Check sheet for the modelled part. Datum: model origin and axes. Units: mm. Coordinates: 2 decimals unless noted, no trailing zeros. Order: outer loops, then holes, each group sorted by start corner. A loop starts at its lowest first (then second) coordinate and runs counter-clockwise, first axis right, second up.
from build123d import *

# Parameters (mm, degrees)
EXTRUDE_1_DEPTH     = 4
SKETCH_3_R          = 2.1
CUT_EXTRUDE_1_DEPTH = 4
SKETCH_4_R          = 10
CUT_EXTRUDE_2_DEPTH = 4
SKETCH_5_W          = 90
SKETCH_5_H          = 5
CUT_EXTRUDE_3_DEPTH = 5
FILLET_1_R          = 5
FILLET_2_R          = 1


with BuildPart() as part:
    # 草图2 → 凸台-拉伸1 (new body)
    with BuildSketch(Plane(origin=(0, 0, 0), x_dir=(1, 0, 0), z_dir=(0, 1, 0))):
        with BuildLine():
            Line((-50, -50), (-50, 50))
            Line((-50, 50), (50, 50))
            Line((50, 50), (50, -50))
            ThreePointArc((50, -50), (0, -100), (-50, -50))
        make_face()
    extrude(amount=EXTRUDE_1_DEPTH)

    # 草图3 → 切除-拉伸1 (cut)
    with BuildSketch(Plane.XZ):
        with Locations(Location((0, 90, 0), (0, 0, 270))):
            Circle(SKETCH_3_R)
        with Locations(Location((43, -43, 0), (0, 0, 270))):
            Circle(SKETCH_3_R)
        with Locations(Location((-43, -43, 0), (0, 0, 270))):
            Circle(SKETCH_3_R)
    extrude(amount=-CUT_EXTRUDE_1_DEPTH, mode=Mode.SUBTRACT)

    # 草图4 → 切除-拉伸2 (cut)
    with BuildSketch(Plane(origin=(0, 4, 0), x_dir=(1, 0, 0), z_dir=(0, 1, 0))):
        with Locations(Location((0, -50, 0), (0, 0, 270))):
            Circle(SKETCH_4_R)
    extrude(amount=-CUT_EXTRUDE_2_DEPTH, mode=Mode.SUBTRACT)

    # 草图5 → 切除-拉伸3 (cut)
    with BuildSketch(Plane(origin=(0, 4, 0), x_dir=(1, 0, 0), z_dir=(0, 1, 0))):
        with Locations((0, 32.5)):
            Rectangle(SKETCH_5_W, SKETCH_5_H)
        with Locations((0, 22.5)):
            Rectangle(SKETCH_5_W, SKETCH_5_H)
        with Locations((0, 12.5)):
            Rectangle(SKETCH_5_W, SKETCH_5_H)
        with Locations((0, 2.5)):
            Rectangle(SKETCH_5_W, SKETCH_5_H)
        with Locations((0, -7.5)):
            Rectangle(SKETCH_5_W, SKETCH_5_H)
        with Locations((0, -17.5)):
            Rectangle(SKETCH_5_W, SKETCH_5_H)
        with Locations((0, -27.5)):
            Rectangle(SKETCH_5_W, SKETCH_5_H)
    extrude(amount=-CUT_EXTRUDE_3_DEPTH, mode=Mode.SUBTRACT)

    # 圆角1
    fillet_1_edges = [part.edges().sort_by_distance(p)[0] for p in [
        (-50, 2, -50),
        (50, 2, -50),
    ]]
    fillet(fillet_1_edges, radius=FILLET_1_R)

    # 圆角2
    fillet_2_edges = [part.edges().sort_by_distance(p)[0] for p in [
        (0, 4, 100),
        (0, 4, -50),
        (-50, 4, 2.5),
        (-48.535533906, 4, -48.535533906),
        (48.535533906, 4, -48.535533906),
        (50, 4, 2.5),
    ]]
    fillet(fillet_2_edges, radius=FILLET_2_R)


solid = part.part
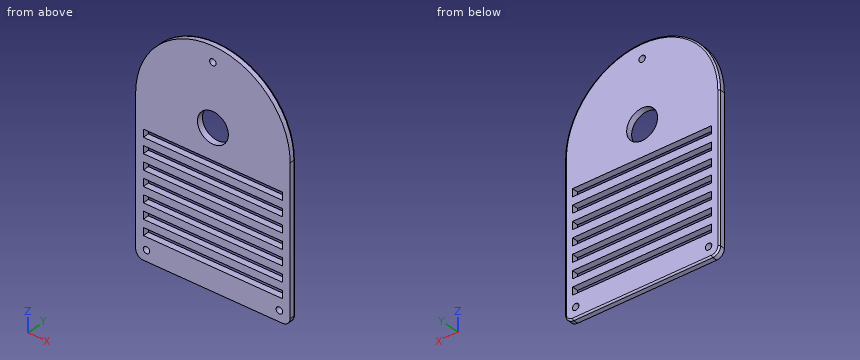
(1) Cross-section at B-B (x = 0). Count the separate pieces of the cut face and the enclosed holes in it, and give its area (3 significant figures).
Filled in:
separate pieces: 10
enclosed holes: 0
area: 363 mm2
(2) Go/stop test with flat-tipped pins: P1, Ø4, axis at x = 43, z = -43, coming from the -Y side; P2, Ø1.2, axis at x = 13.5, y = 1.5, coming from the +Z side. Record where each tip stops, or that it passes through.
Filled in:
P1: passes through
P2: stops at z = 98.31
(3) Cross-section at A-A (z = -43). Enter the section's corners in (x, y).
Filled in:
outline: (-50, 0) - (-45.1, 0) - (-45.1, 4) - (-49, 4) arc R1 ccw to (-50, 3) - close; (-40.9, 0) - (40.9, 0) - (40.9, 4) - (-40.9, 4) - close; (45.1, 0) - (50, 0) - (50, 3) arc R1 ccw to (49, 4) - (45.1, 4) - close
(4) Thickness scan on probe 1 along X at (y, z) = (2.35, -43); probe 2 along X at (y, z) = (1.95, 50); probe 3 along X at (y, z) = (1, 27). Record the ranges inside material, lowest first.
Filled in:
probe 1: x = -50 to -45.1, -40.9 to 40.9, 45.1 to 50
probe 2: x = -50 to -10, 10 to 50
probe 3: x = -50 to -45, 45 to 50
